Build history of the part. All positions in model axes, mm. Face numbers are marked on the shaded views. A direction names the side the tool comes from. Round coordinates to 2 decimals unless told otherwise and drop trailing zeros. Order: outer loops, then holes, each group sorted by start corner. A loop starts at its lowest first (then second) coordinate and runs counter-clockwise, first axis right, second up. Notation, with made-up numbers: (68.25, 20) -> (86.25, 20) arc R26 ccw to (86.25, 53) -> close; hole circle Ø8 at (5.25, 87). An arc over 180 degrees is marked (long way). Answer as a JSON object with one key per item and string values.
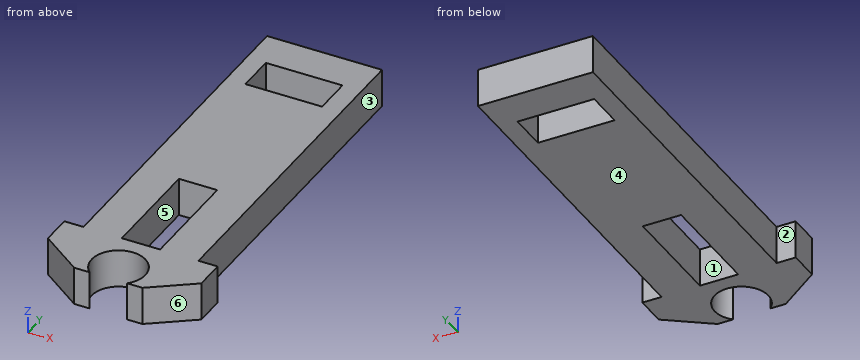
from build123d import *

# Parameters (mm, degrees)
SKETCH1_W           = 5
SKETCH1_H           = 14
SKETCH1_W_2         = 10
SKETCH1_H_2         = 5
BOSS_EXTRUDE1_DEPTH = 5


with BuildPart() as part:
    # Sketch1 → Boss-Extrude1 (new body)
    with BuildSketch(Plane.XY):
        with BuildLine():
            Line((16.949489743, 8), (19.449489743, 8))
            Line((19.449489743, 8), (19.449489743, 4))
            Line((19.449489743, 4), (13.898979486, 0))
            Line((13.898979486, 0), (11.898979486, 0))
            ThreePointArc((11.898979486, 0), (9.449489743, 6), (7, 0))
            Line((7, 0), (5, 0))
            Line((5, 0), (-0.550510257, 4))
            Line((-0.550510257, 4), (-0.550510257, 8))
            Line((-0.550510257, 8), (1.949489743, 8))
            Line((1.949489743, 8), (1.949489743, 53))
            Line((1.949489743, 53), (16.949489743, 53))
            Line((16.949489743, 53), (16.949489743, 8))
        make_face()
        with Locations((9.449489743, 15)):
            Rectangle(SKETCH1_W, SKETCH1_H, mode=Mode.SUBTRACT)
        with Locations((9.449489743, 45.5)):
            Rectangle(SKETCH1_W_2, SKETCH1_H_2, mode=Mode.SUBTRACT)
    extrude(amount=BOSS_EXTRUDE1_DEPTH)


solid = part.part
1) Cut at C-C, the plane z = 2. Give the cut face in (x, y), plus the area to 3 significant figures.
Checked values:
{"outline": "(-0.55, 4) -> (5, 0) -> (7, 0) arc R3.5 cw (long way) to (11.9, 0) -> (13.9, 0) -> (19.45, 4) -> (19.45, 8) -> (16.95, 8) -> (16.95, 53) -> (1.95, 53) -> (1.95, 8) -> (-0.55, 8) -> close; hole (4.45, 43) -> (14.45, 43) -> (14.45, 48) -> (4.45, 48) -> close; hole (6.95, 8) -> (11.95, 8) -> (11.95, 22) -> (6.95, 22) -> close", "area": "658 mm²"}
2) Cut at A-A, the plane y = 16.5. Give the cut face in (x, z).
Checked values:
{"outline": "(1.95, 0) -> (6.95, 0) -> (6.95, 5) -> (1.95, 5) -> close; (11.95, 0) -> (16.95, 0) -> (16.95, 5) -> (11.95, 5) -> close"}
3) Pull direction X, two halves, no side cores. Call the marked faces 4, 5 and 6: pulls with the +X half, pulls with the -X half, needs draft (parallel to the pull), parting line crosses it, or undercut.
Checked values:
{"face 4": "needs draft", "face 5": "undercut", "face 6": "pulls with the +X half"}
4) Cut at B-B, the plane x = 9.25. Give the cut face in (y, z), plus the area to 3 significant figures.
Checked values:
{"outline": "(5.99, 0) -> (8, 0) -> (8, 5) -> (5.99, 5) -> close; (22, 0) -> (43, 0) -> (43, 5) -> (22, 5) -> close; (48, 0) -> (53, 0) -> (53, 5) -> (48, 5) -> close", "area": "140 mm²"}
5) Cut at D-D, the plane y = 2.5. Give the cut face in (x, z), plus the area to 3 significant figures.
Checked values:
{"outline": "(1.53, 0) -> (5.95, 0) -> (5.95, 5) -> (1.53, 5) -> close; (12.95, 0) -> (17.37, 0) -> (17.37, 5) -> (12.95, 5) -> close", "area": "44.2 mm²"}
6) Which spindle directions (+Z, -Z, +X, -X, +Y, -Y) get a long thin tool onto all of the face, cutting with end or side? Do the marked faces 1, 2 and 3. Say none if no direction does.
Checked values:
{"face 1": "+Z, -Z", "face 2": "+Z, -Z, -X, +Y", "face 3": "+Z, -Z, +X, +Y"}
7) Flat gauge pins, fed straight in: pin 1 Ø1.5 at (x, z) = (9.5, 2.5) entering from -Y; pin 2 Ø2 at (x, z) = (19, 2.5) entering from +Y; pin 3 Ø1 at (x, y) = (9.5, 17.5) entering from +Z; pin 4 Ø2.5 at (y, z) = (18, 2.5) entering from +X. Where does each tip first touch, or does it go through?
Checked values:
{"pin 1": "stops at y = 5.91", "pin 2": "stops at y = 8", "pin 3": "passes through", "pin 4": "stops at x = 16.95"}
8) Probe L1, parallel to X at y = 9, z = 1.6; L2, parallel to X at y = 45.5, z = 4.7; L3, parallel to Y at x = 9.5, z = 3.6. List the from-to ranges inside material, lowest first. Write a range as from..to.
Checked values:
{"L1": "x = 1.95..6.95, 11.95..16.95", "L2": "x = 1.95..4.45, 14.45..16.95", "L3": "y = 6..8, 22..43, 48..53"}
